Can you work these out from the model? Positions are in its coordinate system, mm. A direction names the side the tool comes from. Give positions to 0.01 mm unless a question says otherwise; leave off trailing zeros. Order: outer loops, then holes, each group sorted by start corner. A loop starts at its lowest first (then second) coordinate and runs counter-clockwise, first axis right, second up. Notation, with made-up numbers: M 21.5,-37.5 L 52.5,-37.5 A26 cw 52.5,-19.5 Z; hole C 61.25,-12 d1. An arc over 180 degrees is marked long. Write each question's results on one line, items separated by ' | '.
from build123d import *

# Parameters (mm, degrees)
SKETCH1_R           = 1.15
BOSS_EXTRUDE1_DEPTH = 3
SKETCH2_W           = 3
SKETCH2_H           = 25
BOSS_EXTRUDE2_DEPTH = 7
SKETCH3_W           = 15.143900966
SKETCH3_H           = 25
BOSS_EXTRUDE3_DEPTH = 3
SKETCH4_R           = 8.3
CUT_EXTRUDE1_DEPTH  = 1.6
SKETCH5_R           = 2.3
CUT_EXTRUDE2_DEPTH  = 33.480690581
SKETCH6_W           = 3
SKETCH6_H           = 25
BOSS_EXTRUDE4_DEPTH = 10.6
SKETCH7_W           = 28
SKETCH7_H           = 25
SKETCH7_R           = 2.3
SKETCH7_R_2         = 2.5
BOSS_EXTRUDE5_DEPTH = 3


with BuildPart() as part:
    # Sketch1 → Boss-Extrude1 (new body)
    with BuildSketch(Plane(origin=(0, 0, 0), x_dir=(1, 0, 0), z_dir=(0, 1, 0))):
        Polygon((12.5, 12.5), (-12.5, 12.5), (-12.5, -12.5), (12.5, -12.5), (15.5, -12.5), (15.5, 12.5), align=None)
        with Locations(Location((-7.7, 7.7, 0), (0, 0, 270))):
            Circle(SKETCH1_R, mode=Mode.SUBTRACT)
        with Locations(Location((-7.7, -7.7, 0), (0, 0, 270))):
            Circle(SKETCH1_R, mode=Mode.SUBTRACT)
        with Locations(Location((7.7, -7.7, 0), (0, 0, 270))):
            Circle(SKETCH1_R, mode=Mode.SUBTRACT)
        with Locations(Location((7.7, 7.7, 0), (0, 0, 270))):
            Circle(SKETCH1_R, mode=Mode.SUBTRACT)
    extrude(amount=BOSS_EXTRUDE1_DEPTH)

    # Sketch2 → Boss-Extrude2 (add)
    with BuildSketch(Plane(origin=(0, 3, 0), x_dir=(1, 0, 0), z_dir=(0, 1, 0))):
        with Locations((14, 0)):
            Rectangle(SKETCH2_W, SKETCH2_H)
    extrude(amount=BOSS_EXTRUDE2_DEPTH)

    # Sketch3 → Boss-Extrude3 (add)
    with BuildSketch(Plane(origin=(0, 10, 0), x_dir=(1, 0, 0), z_dir=(0, 1, 0))):
        with Locations((20.071950483, 0)):
            Rectangle(SKETCH3_W, SKETCH3_H)
    extrude(amount=BOSS_EXTRUDE3_DEPTH)

    # Sketch4 → Cut-Extrude1 (cut)
    with BuildSketch(Plane(origin=(0, 3, 0), x_dir=(1, 0, 0), z_dir=(0, 1, 0))):
        with Locations(Location((0, 0, 0), (0, 0, 270))):
            Circle(SKETCH4_R)
    extrude(amount=-CUT_EXTRUDE1_DEPTH, mode=Mode.SUBTRACT)

    # Sketch5 → Cut-Extrude2 (cut, through all)
    with BuildSketch(Plane(origin=(0, 1.4, 0), x_dir=(1, 0, 0), z_dir=(0, 1, 0))):
        with Locations(Location((0, 0, 0), (0, 0, 270))):
            Circle(SKETCH5_R)
    extrude(amount=-CUT_EXTRUDE2_DEPTH, mode=Mode.SUBTRACT)

    # Sketch6 → Boss-Extrude4 (add)
    with BuildSketch(Plane.XZ):
        with Locations((14, 0)):
            Rectangle(SKETCH6_W, SKETCH6_H)
    extrude(amount=BOSS_EXTRUDE4_DEPTH)

    # Sketch7 → Boss-Extrude5 (add)
    with BuildSketch(Plane.XZ.offset(10.6)):
        with Locations((1.5, 0)):
            Rectangle(SKETCH7_W, SKETCH7_H)
        with Locations(Location((0, 0, 0), (0, 0, 90))):
            Circle(SKETCH7_R, mode=Mode.SUBTRACT)
        with Locations(Location((-7.7, 7.7, 0), (0, 0, 270))):
            Circle(SKETCH7_R_2, mode=Mode.SUBTRACT)
        with Locations(Location((-7.7, -7.7, 0), (0, 0, 270))):
            Circle(SKETCH7_R_2, mode=Mode.SUBTRACT)
        with Locations(Location((7.7, -7.7, 0), (0, 0, 270))):
            Circle(SKETCH7_R_2, mode=Mode.SUBTRACT)
        with Locations(Location((7.7, 7.7, 0), (0, 0, 270))):
            Circle(SKETCH7_R_2, mode=Mode.SUBTRACT)
    extrude(amount=BOSS_EXTRUDE5_DEPTH)


solid = part.part
(1) We'd pull the mould along Y, two halves only. Please class faces 1 (the face through (12.5, -5, 0)), 2 (the face through (-12.5, -12, 0)), 3 (the face through (20, 13, 0)), 4 (the face through (21, 10, 0)): +Y half, -Y half, draft (parallel to the pull), parting line (faces both ways), or undercut.
Data:
face 1: undercut | face 2: draft | face 3: +Y half | face 4: -Y half
(2) Imagine slicing it at C-C, the plane x = -7.7. Write out the boundary of the cut face in (y, z), plus the area to 3 significant figures.
Data:
outline: M -13.6,-12.5 L -10.6,-12.5 L -10.6,-10.2 L -13.6,-10.2 Z; M -13.6,-5.2 L -10.6,-5.2 L -10.6,5.2 L -13.6,5.2 Z; M -13.6,10.2 L -10.6,10.2 L -10.6,12.5 L -13.6,12.5 Z; M 0,-12.5 L 3,-12.5 L 3,-8.85 L 0,-8.85 Z; M 0,-6.55 L 3,-6.55 L 3,-3.1 L 1.4,-3.1 L 1.4,3.1 L 3,3.1 L 3,6.55 L 0,6.55 Z; M 0,8.85 L 3,8.85 L 3,12.5 L 0,12.5 Z | area: 96.3 mm2
(3) Imagine slicing it at A-A, the plane x = 0. Write out the boundary of the cut face in (y, z), plus the area to 3 significant figures.
Data:
outline: M -13.6,-12.5 L -10.6,-12.5 L -10.6,-2.3 L -13.6,-2.3 Z; M -13.6,2.3 L -10.6,2.3 L -10.6,12.5 L -13.6,12.5 Z; M 0,-12.5 L 3,-12.5 L 3,-8.3 L 1.4,-8.3 L 1.4,-2.3 L 0,-2.3 Z; M 0,2.3 L 1.4,2.3 L 1.4,8.3 L 3,8.3 L 3,12.5 L 0,12.5 Z | area: 103 mm2
(4) I need wall thicknesses on L1, parallel to X at y = -11.6, z = -7.7; L2, parallel to Y at x = 5, z = 7; L3, parallel to X at y = 1.1, z = 0. Which ranges of each line are inside material? Lowest first, please. Write a range as from..to.
Data:
L1: x = -12.5..-10.2, -5.2..5.2, 10.2..15.5 | L2: y = -13.6..-10.6, 0..3 | L3: x = -12.5..-2.3, 2.3..15.5
(5) Imagine slicing it at B-B, the plane z = 0. Write out the boundary of the cut face in (x, y), plus the area to 3 significant figures.
Data:
outline: M -12.5,-13.6 L -2.3,-13.6 L -2.3,-10.6 L -12.5,-10.6 Z; M -12.5,0 L -2.3,0 L -2.3,1.4 L -8.3,1.4 L -8.3,3 L -12.5,3 Z; M 2.3,-13.6 L 15.5,-13.6 L 15.5,10 L 27.64,10 L 27.64,13 L 12.5,13 L 12.5,3 L 8.3,3 L 8.3,1.4 L 2.3,1.4 L 2.3,0 L 12.5,0 L 12.5,-10.6 L 2.3,-10.6 Z | area: 219 mm2
(6) Will these pins go through, and if not, where does the flat tip stop? P1, Ø8, axis at y = -1, z = -5, coming from the +X side; P2, Ø3, axis at x = -7.7, z = 7.7, coming from the +Y side; P3, Ø13.5, axis at x = 0, z = 0, coming from the +Y side.
Data:
P1: stops at x = 15.5 | P2: stops at y = 3 | P3: stops at y = 1.4
(7) Imagine slicing it at D-D, the plane z = 7.7. Count the separate pieces of the cut face and the enclosed holes in it, plus the area to 3 significant figures.
Data:
separate pieces: 5 | enclosed holes: 0 | area: 213 mm2
(8) For faces 5 (the face through (-5.05, 2.211, -6.587)), 6 (the face through (12.5, 8, 0)), 7 (the face through (-5.59, -12.08, -9.04)), 8 (the face through (15.5, -2, 0)), which set-ups out of +Z, -Z, +X, -X, +Y, -Y let a thin tool reach every point of the face, with its end or its side?
Data:
face 5: +Y | face 6: +Z, -Z, -X, +Y | face 7: -Y | face 8: +Z, -Z, +X, -Y
